For this review, take the finished solid that the model builds, in its own axes (mm). A direction names the side the tool comes from. Coordinates: 2 decimals unless noted, no trailing zeros. Loops run counter-clockwise (first coordinate to the right, second up) from the corner with the lowest first, then second, coordinate; pieces in that order, holes last. Notation, with made-up numbers: (63.5, -38.75) - (117.5, -38.75) arc R23 cw to (117.5, -18.75) - close; hole circle Ø5 at (23.5, 78.25). An arc over 180 degrees is marked (long way). One line per item, written item: value. Start each with the question number.
1. To check wall thickness, follow line 1 (Y direction, x = 0, z = -0.5); line 2 (Z direction, x = -3.25, y = 3.8); line 3 (X direction, y = -0.2, z = -0.2). State the ranges of each line that lie inside material, in increasing order. Write a range as from..to.
2. Take a section at A-A, the plane x = 0. State the section outline as (y, z) points, and give its area (3 significant figures).
3. Insertion check: pin 1 (1.4 mm diameter, centred on x = -1.5, y = 2, fed in from -Z); pin 2 (0.5 mm diameter, centred on x = 4, y = -0.5, fed in from -Z); pin 3 (0.7 mm diameter, centred on x = 2, y = -0.5, fed in from +Z). Each pin has a flat end and moves straight along its axis. Give the tip position at first contact, or say it passes through.
4. Take a section at B-B, the plane x = 3.98. State the section outline as (y, z) points, and give its area (4 significant figures).
5. For faces 1 (the face through (-0.28, -1.27, 0.01)), 2 (the face through (4, -1, 0.7)), 3 (the face through (-3.467, 1.604, 0.008)), list the 3-axis set-ups (+Z, -Z, +X, -X, +Y, -Y) from which the entire face can be reached by the end or side of a thin tool; tool diameter is ignored.
```python
from build123d import *

# Parameters (mm, degrees)
SKETCH1_R           = 1.3
SKETCH1_R_2         = 0.3
BOSS_EXTRUDE1_DEPTH = 1
SKETCH1_3_R         = 0.7625
BOSS_EXTRUDE2_DEPTH = 0.7
BOSS_EXTRUDE3_DEPTH = 0.6
BOSS_EXTRUDE4_DEPTH = 0.6
BOSS_EXTRUDE5_DEPTH = 0.4
SKETCH5_R           = 0.3
BOSS_EXTRUDE6_DEPTH = 0.4


with BuildPart() as part:
    # Sketch1 → Boss-Extrude1 (new body, symmetric)
    with BuildSketch(Plane.XY):
        Circle(SKETCH1_R)
        Circle(SKETCH1_R_2, mode=Mode.SUBTRACT)
    extrude(amount=BOSS_EXTRUDE1_DEPTH, both=True)



with BuildPart() as body_2:
    # Sketch1_3 → Boss-Extrude2 (new body, symmetric)
    with BuildSketch(Plane.XY):
        with Locations((3.98, -0.66624549)):
            Circle(SKETCH1_3_R)
    extrude(amount=BOSS_EXTRUDE2_DEPTH, both=True)


with BuildPart() as part_1:
    add(part.part)

    add(body_2.part)  # Boss-Extrude3 merges body 2
    # Sketch1_4 → Boss-Extrude3 (add, symmetric)
    with BuildSketch(Plane.XY):
        with BuildLine():
            ThreePointArc((3.374350994, -1.12949006), (3.252423356, -0.438126053), (3.747253005, 0.059864065))
            Line((3.747253005, 0.059864065), (2.019976925, 1.088093316))
            Line((2.019976925, 1.088093316), (0.140477621, 1.292387727))
            ThreePointArc((0.140477621, 1.292387727), (0.967631362, 0.868152951), (1.3, 0))
            ThreePointArc((1.3, 0), (1.183953974, -0.536891971), (0.856533864, -0.977931357))
            add(Edge.make_bspline(
                [(3.374350994, -1.12949006), (2.778476345, -0.90659845), (2.406966993, -0.786012749), (1.50197992, -0.807474496), (0.996483155, -0.855354956), (0.856533864, -0.977931357)],
                knots=[0, 0, 0, 0, 0.647248286, 0.718239717, 1, 1, 1, 1], degree=3))
        make_face()
    extrude(amount=BOSS_EXTRUDE3_DEPTH, both=True)

    # Sketch1_5 → Boss-Extrude4 (add, symmetric)
    with BuildSketch(Plane.XY):
        with BuildLine():
            ThreePointArc((-1.295848634, -0.103809043), (-1.071749439, 0.735767042), (-0.368782161, 1.24659525))
            Line((-0.368782161, 1.24659525), (-2.254212966, 2.57050074))
            Line((-2.254212966, 2.57050074), (-3.469420101, 2.791170079))
            Line((-3.469420101, 2.791170079), (-3.851452989, 2.234684794))
            Line((-3.851452989, 2.234684794), (-3.20884425, 1.179944376))
            Line((-3.20884425, 1.179944376), (-1.295848634, -0.103809043))
        make_face()
    extrude(amount=BOSS_EXTRUDE4_DEPTH, both=True)



with BuildPart() as body_2_2:
    # Sketch2 → Revolve1 (revolve)
    with BuildSketch(Plane.XY):
        with BuildLine():
            Line((-3.851452989, 2.234684794), (-3.357165564, 2.954684794))
            Line((-3.357165564, 2.954684794), (-3.682812508, 3.17824478))
            Line((-3.682812508, 3.17824478), (-4.833144721, 1.502622153))
            ThreePointArc((-4.833144721, 1.502622153), (-4.406042562, 1.526493017), (-4.321028806, 1.945728909))
            Line((-4.321028806, 1.945728909), (-3.851452989, 2.234684794))
        make_face()
    revolve(axis=Axis((-3.682812508, 3.17824478, 0), (-0.565974648, -0.824422645, 0)))


with BuildPart() as part_2:
    add(part_1.part)

    add(body_2_2.part)  # Revolve2 merges body 2 2
    # Sketch3 → Revolve2 (revolve)
    with BuildSketch(Plane.XY):
        Polygon((-3.62534147, 3.261959529), (-4.236594089, 2.371583072), (-4.986818697, 2.886620001), (-4.375566077, 3.776996458), align=None)
    revolve(axis=Axis((-3.62534147, 3.261959529, 0), (-0.565974648, -0.824422645, 0)))

    # Sketch4 → Boss-Extrude5 (add)
    with BuildSketch(Plane(origin=(0.36074202, 0.525472106, 0), x_dir=(0.824422645, -0.565974648, 0), z_dir=(0.565974648, 0.824422645, 0))):
        Polygon((-4.835, -0.75055535), (-4.185, -0.375277675), (-4.185, 0.375277675), (-4.835, 0.75055535), (-5.485, 0.375277675), (-5.485, -0.375277675), align=None)
    extrude(amount=BOSS_EXTRUDE5_DEPTH)

    # Sketch5 → Boss-Extrude6 (add)
    with BuildSketch(Plane(origin=(0.587131879, 0.855241165, 0), x_dir=(0.824422645, -0.565974648, 0), z_dir=(0.565974648, 0.824422645, 0))):
        with Locations((-4.835, 0)):
            Circle(SKETCH5_R)
    extrude(amount=BOSS_EXTRUDE6_DEPTH)


solid = part_2.part
```
Solutions:
1. line 1: -1.3..-0.3, 0.3..1.3
1. line 2: -0.3..0.3
1. line 3: -1.28..-0.22, 0.22..4.58
2. outline: (-1.3, -1) - (-0.3, -1) - (-0.3, 1) - (-1.3, 1) - close; (0.3, -1) - (1.3, -1) - (1.3, 1) - (0.3, 1) - close
2. area: 4.00 mm2
3. pin 1: z = -0.6
3. pin 2: z = -0.7
3. pin 3: z = 0.6
4. outline: (-1.43, -0.7) - (0.1, -0.7) - (0.1, 0.7) - (-1.43, 0.7) - close
4. area: 2.135 mm2
5. face 1: none
5. face 2: +Z, +X, +Y, -Y
5. face 3: +Z, -Z, -Y
